Check sheet for the modelled part. Datum: model origin and axes. Units: mm. A direction names the side the tool comes from. Round coordinates to 2 decimals unless told otherwise and drop trailing zeros. Write each loop counter-clockwise with the first axis right and the second up, starting at its lowest first coordinate (ties: lowest second). Pieces come first, ordered by that corner, then holes. Notation, with made-up numbers: M 72.5,66 L 125.5,66 A17 ccw 125.5,90 Z; hole C -37.75,63.25 d1. An arc over 180 degrees is marked long. Put each result on its own line as item: value.
```python
from build123d import *

# Parameters (mm, degrees)
ESBO_O1_W                = 113
ESBO_O1_H                = 26.5
RESSALTO_EXTRUS_O1_DEPTH = 5
ESBO_O2_W                = 5
ESBO_O2_H                = 7.62
CORTE_EXTRUS_O1_DEPTH    = 5
CORTE_EXTRUS_O2_DEPTH    = 5
CORTE_EXTRUS_O3_DEPTH    = 10


with BuildPart() as part:
    # Esboço1 → Ressalto-extrusão1 (new body)
    with BuildSketch(Plane(origin=(0, 0, 0), x_dir=(1, 0, 0), z_dir=(0, 1, 0))):
        with Locations((-20.23644711, -18.909257917)):
            Rectangle(ESBO_O1_W, ESBO_O1_H)
    extrude(amount=RESSALTO_EXTRUS_O1_DEPTH)

    # Esboço2 → Corte-extrusão1 (cut)
    with BuildSketch(Plane(origin=(0, 5, 0), x_dir=(1, 0, 0), z_dir=(0, 1, 0))):
        with Locations((13.76355289, -18.914257917)):
            Rectangle(ESBO_O2_W, ESBO_O2_H)
        with Locations((-54.23644711, -18.914257917)):
            Rectangle(ESBO_O2_W, ESBO_O2_H)
    extrude(amount=-CORTE_EXTRUS_O1_DEPTH, mode=Mode.SUBTRACT)

    # Esboço3 → Corte-extrusão2 (cut)
    with BuildSketch(Plane(origin=(0, 5, 0), x_dir=(1, 0, 0), z_dir=(0, 1, 0))):
        Polygon((-76.73644711, -17.909257917), (-73.23644711, -17.909257917), (-73.23644711, -16.109257917), (-71.73644711, -16.109257917), (-71.73644711, -17.909257917), (-69.73644711, -17.909257917), (-69.73644711, -19.909257917), (-71.73644711, -19.909257917), (-71.73644711, -21.709257917), (-73.23644711, -21.709257917), (-73.23644711, -19.909257917), (-76.73644711, -19.909257917), align=None)
        Polygon((-51.73644711, -17.909257917), (-48.23644711, -17.909257917), (-48.23644711, -16.109257917), (-46.73644711, -16.109257917), (-46.73644711, -17.909257917), (-44.73644711, -17.909257917), (-44.73644711, -19.909257917), (-46.73644711, -19.909257917), (-46.73644711, -21.709257917), (-48.23644711, -21.709257917), (-48.23644711, -19.909257917), (-51.73644711, -19.909257917), align=None)
    corte_extrus_o2 = extrude(amount=-CORTE_EXTRUS_O2_DEPTH, mode=Mode.SUBTRACT)

    # Espelhar1: Corte-extrusão2 across plane
    add(corte_extrus_o2.mirror(Plane.ZY.offset(20.23644711)), mode=Mode.SUBTRACT)

    # Esboço4 → Corte-extrusão3 (cut)
    with BuildSketch(Plane.XZ):
        with BuildLine():
            Line((-4.73644711, 13.909257917), (-35.73644711, 13.909257917))
            ThreePointArc((-35.73644711, 13.909257917), (-37.150660672, 14.495044355), (-37.73644711, 15.909257917))
            Line((-37.73644711, 15.909257917), (-37.73644711, 21.909257917))
            ThreePointArc((-37.73644711, 21.909257917), (-37.150660672, 23.32347148), (-35.73644711, 23.909257917))
            Line((-35.73644711, 23.909257917), (-4.73644711, 23.909257917))
            ThreePointArc((-4.73644711, 23.909257917), (-3.322233548, 23.32347148), (-2.73644711, 21.909257917))
            Line((-2.73644711, 21.909257917), (-2.73644711, 15.909257917))
            ThreePointArc((-2.73644711, 15.909257917), (-3.322233548, 14.495044355), (-4.73644711, 13.909257917))
        make_face()
    extrude(amount=-CORTE_EXTRUS_O3_DEPTH, mode=Mode.SUBTRACT)


solid = part.part
```
1. Cross-section at B-B (x = -34.5). Enter the section's corners in (y, z), then the cut area to 3 significant figures.
Computed values:
outline: M 0,5.66 L 5,5.66 L 5,13.91 L 0,13.91 Z; M 0,23.91 L 5,23.91 L 5,32.16 L 0,32.16 Z
area: 82.5 mm2
2. Scan lines: probe 1 along X at (y, z) = (1.2, 18.25); probe 2 along X at (y, z) = (3.95, 16); probe 3 along Z at (x, y) = (12, 3.5). Record each from-to range of solid material in increasing order.
Computed values:
probe 1: x = -69.74 to -56.74, -44.74 to -37.74, -2.74 to 4.26, 16.26 to 29.26
probe 2: x = -76.74 to -56.74, -51.74 to -37.74, -2.74 to 11.26, 16.26 to 36.26
probe 3: z = 5.66 to 15.1, 22.72 to 32.16
3. Depth check by flat-ended pin: pin 1 Ø0.6 at (y, z) = (3.5, 19) entering from -X. Enter the tip coordinate at first touch or a pass-through.
Computed values:
pin 1: stops at x = -69.74
4. Release check for a two-part mould opening along X. For faces 4 (the flat face through (-44.736, 3, 19)), 5 (the flat face through (-76.736, 2, 12)), 6 (the flat face through (35, 3, 17.909)) record: +X half, -X half, draft (parallel to the pull), parting line (faces both ways), or undercut.
Computed values:
face 4: undercut
face 5: -X half
face 6: draft
5. Cross-section at C-C (y = 1.6). Count the separate pieces of the cut face and the enclosed holes in it, then the cut area to 3 significant figures.
Computed values:
separate pieces: 1
enclosed holes: 3
area: 2,490 mm2
6. Cross-section at A-A (x = -54.5). Enter the section's corners in (y, z).
Computed values:
outline: M 0,5.66 L 5,5.66 L 5,15.1 L 0,15.1 Z; M 0,22.72 L 5,22.72 L 5,32.16 L 0,32.16 Z
7. Access from +Z, -Z, +X, -X, +Y, -Y to the whole of each face (thin tool, end or side, straight path). Record for faces 1 (the flat face through (-75, 3, 17.909)), 2 (the flat face through (-21, 2, 5.659)), 3 (the flat face through (-71.736, 3, 21)).
Computed values:
face 1: -X, +Y, -Y
face 2: -Z, +X, -X, +Y, -Y
face 3: +Y, -Y
